from build123d import *

# Parameters (mm, degrees)
SKETCH1_W                = 290
SKETCH1_H                = 16
BOSS_EXTRUDE1_DEPTH      = 12.5
M5_TAPPED_HOLE1_D        = 4.2
SKETCH7_W                = 25
SKETCH7_H                = 24.547818694
CUT_EXTRUDE2_DEPTH       = 147.414650906
CHAMFER1_SIZE            = 2
CHAMFER1_OF_MIRROR1_SIZE = 2
G1_8_TAPPED_HOLE1_D      = 8.8
G1_8_TAPPED_HOLE1_DEPTH  = 9
G1_8_TAPPED_HOLE1_TIP    = 2.643786724
M6_TAPPED_HOLE1_D        = 5
M6_TAPPED_HOLE1_DEPTH    = 15
M6_TAPPED_HOLE1_TIP      = 1.502151548


with BuildPart() as part:
    # Sketch1 → Boss-Extrude1 (new, symmetric)
    with BuildSketch(Plane(origin=(0, 0, 0), x_dir=(1, 0, 0), z_dir=(0, 1, 0))):
        Rectangle(SKETCH1_W, SKETCH1_H)
    extrude(amount=BOSS_EXTRUDE1_DEPTH, both=True)

    # M5 Tapped Hole1 (through all)
    with Locations(Plane(origin=(0, 12.5, 0), x_dir=(1, 0, 0), z_dir=(0, 1, 0))):
        with Locations((-110, 0), (110, 0)):
            Hole(M5_TAPPED_HOLE1_D / 2)

    # Sketch7 → Cut-Extrude2 (cut, through all)
    with BuildSketch(Plane.XY.offset(8)):
        with Locations((110, -14.273909347)):
            Rectangle(SKETCH7_W, SKETCH7_H)
    cut_extrude2 = extrude(amount=-CUT_EXTRUDE2_DEPTH, mode=Mode.SUBTRACT)

    # Chamfer1
    chamfer1_edges = [part.edges().sort_by_distance(p)[0] for p in [
        (122.5, -12.5, 0),
        (97.5, -12.5, 0),
    ]]
    chamfer(chamfer1_edges, length=CHAMFER1_SIZE)

    # Mirror1: Cut-Extrude2 across plane
    add(cut_extrude2.mirror(Plane(origin=(0, 0, 0), x_dir=(0, 0, 1), z_dir=(1, 0, 0))), mode=Mode.SUBTRACT)

    # Chamfer1 of Mirror1
    chamfer1_of_mirror1_edges = [part.edges().sort_by_distance(p)[0] for p in [
        (-122.5, -12.5, 0),
        (-97.5, -12.5, 0),
    ]]
    chamfer(chamfer1_of_mirror1_edges, length=CHAMFER1_OF_MIRROR1_SIZE)

    # G1/8 Tapped Hole1
    with Locations(Plane(origin=(0, 12.5, 0), x_dir=(1, 0, 0), z_dir=(0, 1, 0))):
        with Locations((-110, 0), (110, 0)):
            Hole(G1_8_TAPPED_HOLE1_D / 2, depth=G1_8_TAPPED_HOLE1_DEPTH)
            with Locations((0, 0, -(G1_8_TAPPED_HOLE1_DEPTH + G1_8_TAPPED_HOLE1_TIP / 2))):  # 118° drill point
                Cone(0, G1_8_TAPPED_HOLE1_D / 2, G1_8_TAPPED_HOLE1_TIP, mode=Mode.SUBTRACT)

    # M6 Tapped Hole1
    with Locations(Plane(origin=(0, 12.5, 0), x_dir=(1, 0, 0), z_dir=(0, 1, 0))):
        with Locations((-140, 0), (-127.5, 0), (127.5, 0), (140, 0)):
            Hole(M6_TAPPED_HOLE1_D / 2, depth=M6_TAPPED_HOLE1_DEPTH)
            with Locations((0, 0, -(M6_TAPPED_HOLE1_DEPTH + M6_TAPPED_HOLE1_TIP / 2))):  # 118° drill point
                Cone(0, M6_TAPPED_HOLE1_D / 2, M6_TAPPED_HOLE1_TIP, mode=Mode.SUBTRACT)


solid = part.part
The listing builds one solid part. Answer for the finished solid, in the listing's coordinates (mm). A direction names the side the tool comes from. Round coordinates to 2 decimals unless told otherwise and drop trailing zeros. Write each question's results on one line, items separated by ' | '. Start each with the question number.
(1) Find the intervals of material crossed by line 1 (X direction, y = -4, z = -5); line 2 (Z direction, x = -140, y = 1); line 3 (X direction, y = 4.5, z = -3.5), in increasing order.
(2) Determine the mould class of faces 1 (the cylindrical face through (-142.385, 4.895, -0.751)), 2 (the flat face through (-2, 0, -8)), 3 (the flat face through (-1, -12.5, 0)) for opening direction Z: +Z half, -Z half, draft (parallel to the pull), parting line (faces both ways), or undercut.
(3) Each of these flat-tipped pins is pushed along its axis until it touches: P1, Ø5, axis at x = 110, z = 0, coming from the +Y side; P2, Ø4.5, axis at x = 140, z = 0, coming from the +Y side; P3, Ø3, axis at x = -127.5, z = 0, coming from the +Y side. Where does it stop, or does it pass through?
(4) For faces 4 (the flat face through (-97.5, -6, 0)), 5 (the cylindrical face through (-129.885, 4.895, -0.751)), 6 (the flat face through (-135, -12.5, 0)), determine the directions among +Z, -Z, +X, -X, +Y, -Y from which every point of the face is accessible in a straight line to the end or side of a thin tool.
Worked answers:
1) line 1: x = -145 to -122.5, -97.5 to 97.5, 122.5 to 145 | line 2: z = -8 to -2.5, 2.5 to 8 | line 3: x = -145 to -112.67, -107.33 to 107.33, 112.67 to 145
2) face 1: undercut | face 2: -Z half | face 3: draft
3) P1: stops at y = 2.36 | P2: stops at y = -2.65 | P3: stops at y = -3.1
4) face 4: +Z, -Z, -Y | face 5: +Y | face 6: +Z, -Z, +X, -X, -Y
